Work out the finished part from the listing and answer in its coordinate system (mm). Face numbers are marked on the shaded views. A direction names the side the tool comes from. Coordinates: 2 decimals unless noted, no trailing zeros. Order: outer loops, then holes, each group sorted by start corner. A loop starts at its lowest first (then second) coordinate and runs counter-clockwise, first axis right, second up.
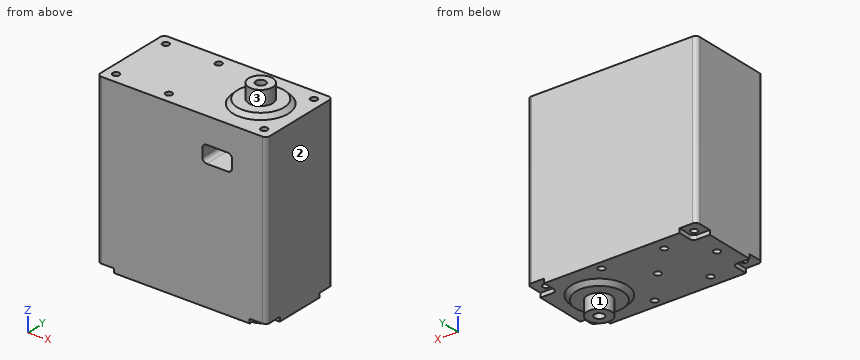
```python
from build123d import *

# Parameters (mm, degrees)
ESQUISSE1_W             = 40
ESQUISSE1_H             = 20
BOSS_EXTRU_1_DEPTH      = 40.5
ESQUISSE2_R             = 0.79
ENL_V_MAT_EXTRU_2_DEPTH = 61.334484335
ENL_V_MAT_EXTRU_3_DEPTH = 1
ESQUISSE4_R             = 0.79
ENL_V_MAT_EXTRU_4_DEPTH = 20
ESQUISSE5_R             = 6.5
BOSS_EXTRU_2_DEPTH      = 1
CHANFREIN1_SIZE         = 1
ESQUISSE6_R             = 2.85
BOSS_EXTRU_3_DEPTH      = 3.4
CONG_1_R                = 1
BOSS_EXTRU_4_START      = 1
ESQUISSE7_R             = 6.5
BOSS_EXTRU_4_DEPTH      = 1
CHANFREIN2_SIZE         = 1
BOSS_EXTRU_5_START      = 3.4
ESQUISSE8_R             = 2.85
BOSS_EXTRU_5_DEPTH      = 3.4
ENL_V_MAT_EXTRU_6_DEPTH = 15
ESQUISSE10_R            = 0.79
ENL_V_MAT_EXTRU_7_DEPTH = 20
ESQUISSE11_R            = 1.15
ENL_V_MAT_EXTRU_8_DEPTH = 15
ENL_V_START             = -15
ESQUISSE12_R            = 1.15
ENL_V_MAT_EXTRU_9_DEPTH = 15


with BuildPart() as part:
    # Esquisse1 → Boss.-Extru.1 (new body)
    with BuildSketch(Plane.XY):
        with Locations((20, 10)):
            Rectangle(ESQUISSE1_W, ESQUISSE1_H)
    extrude(amount=BOSS_EXTRU_1_DEPTH)

    # Esquisse2 → Enlèv. mat.-Extru.2 (cut, through all)
    with BuildSketch(Plane(origin=(0, 0, 0), x_dir=(-1, 0, 0), z_dir=(0, 0, -1))):
        with Locations((-2.5, 2.5)):
            Circle(ESQUISSE2_R)
        with Locations((-37.5, 2.5)):
            Circle(ESQUISSE2_R)
        with Locations((-2.5, 17.5)):
            Circle(ESQUISSE2_R)
        with Locations((-37.5, 17.5)):
            Circle(ESQUISSE2_R)
    extrude(amount=-ENL_V_MAT_EXTRU_2_DEPTH, mode=Mode.SUBTRACT)

    # Esquisse3 → Enlèv. mat.-Extru.3 (cut)
    with BuildSketch(Plane(origin=(0, 0, 0), x_dir=(-1, 0, 0), z_dir=(0, 0, -1))):
        with BuildLine():
            Line((0, 16), (-3, 16))
            ThreePointArc((-3, 16), (-3.707106781, 16.292893219), (-4, 17))
            Line((-4, 17), (-4, 20))
            Line((-4, 20), (0, 20))
            Line((0, 20), (0, 16))
        make_face()
        with BuildLine():
            Line((0, 0), (-4, 0))
            Line((-4, 0), (-4, 3))
            ThreePointArc((-4, 3), (-3.707106781, 3.707106781), (-3, 4))
            Line((-3, 4), (0, 4))
            Line((0, 4), (0, 0))
        make_face()
        with BuildLine():
            Line((-36, 0), (-40, 0))
            Line((-40, 0), (-40, 4))
            Line((-40, 4), (-37, 4))
            ThreePointArc((-37, 4), (-36.292893219, 3.707106781), (-36, 3))
            Line((-36, 3), (-36, 0))
        make_face()
        with BuildLine():
            Line((-37, 16), (-40, 16))
            Line((-40, 16), (-40, 20))
            Line((-40, 20), (-36, 20))
            Line((-36, 20), (-36, 17))
            ThreePointArc((-36, 17), (-36.292893219, 16.292893219), (-37, 16))
        make_face()
    extrude(amount=-ENL_V_MAT_EXTRU_3_DEPTH, mode=Mode.SUBTRACT)

    # Esquisse4 → Enlèv. mat.-Extru.4 (cut)
    with BuildSketch(Plane(origin=(0, 0, 0), x_dir=(-1, 0, 0), z_dir=(0, 0, -1))):
        with Locations((-3, 10)):
            Circle(ESQUISSE4_R)
        with Locations((-10, 17)):
            Circle(ESQUISSE4_R)
        with Locations((-10, 3)):
            Circle(ESQUISSE4_R)
        with Locations((-17, 10)):
            Circle(ESQUISSE4_R)
        with Locations((-24, 2)):
            Circle(ESQUISSE4_R)
        with Locations((-24, 18)):
            Circle(ESQUISSE4_R)
    extrude(amount=-ENL_V_MAT_EXTRU_4_DEPTH, mode=Mode.SUBTRACT)

    # Esquisse5 → Boss.-Extru.2 (add)
    with BuildSketch(Plane(origin=(0, 0, 0), x_dir=(-1, 0, 0), z_dir=(0, 0, -1))):
        with Locations((-30.8, 10)):
            Circle(ESQUISSE5_R)
    extrude(amount=BOSS_EXTRU_2_DEPTH)

    # Chanfrein1
    chanfrein1_edges = [part.edges().sort_by_distance(p)[0] for p in [
        (37.3, 10, -1),
    ]]
    chamfer(chanfrein1_edges, length=CHANFREIN1_SIZE - 0.0001)  # a hair under: the kernel refuses the full size

    # Esquisse6 → Boss.-Extru.3 (add)
    with BuildSketch(Plane(origin=(0, 0, -1), x_dir=(-1, 0, 0), z_dir=(0, 0, -1))):
        with Locations((-30.8, 10)):
            Circle(ESQUISSE6_R)
    extrude(amount=BOSS_EXTRU_3_DEPTH)

    # Congé1
    cong_1_edges = [part.edges().sort_by_distance(p)[0] for p in [
        (0, 20, 20.75),
        (40, 20, 20.75),
        (40, 0, 20.75),
        (0, 0, 20.75),
    ]]
    fillet(cong_1_edges, radius=CONG_1_R)

    # Esquisse7 → Boss.-Extru.4 (add)
    with BuildSketch(Plane.XY.offset(40.5).offset(BOSS_EXTRU_4_START)):
        with Locations(Location((30.8, 10, 0), (0, 0, 180))):
            Circle(ESQUISSE7_R)
    extrude(amount=-BOSS_EXTRU_4_DEPTH)

    # Chanfrein2
    chanfrein2_edges = [part.edges().sort_by_distance(p)[0] for p in [
        (37.3, 10, 41.5),
    ]]
    chamfer(chanfrein2_edges, length=CHANFREIN2_SIZE - 0.0001)  # a hair under: the kernel refuses the full size

    # Esquisse8 → Boss.-Extru.5 (add)
    with BuildSketch(Plane.XY.offset(41.5).offset(BOSS_EXTRU_5_START)):
        with Locations(Location((30.8, 10, 0), (0, 0, 180))):
            Circle(ESQUISSE8_R)
    extrude(amount=-BOSS_EXTRU_5_DEPTH)

    # Esquisse9 → Enlèv. mat.-Extru.6 (cut)
    with BuildSketch(Plane.XZ):
        with BuildLine():
            Line((30.852193658, 30.389388186), (25.852193658, 30.389388186))
            ThreePointArc((25.852193658, 30.389388186), (25.145086877, 30.682281405), (24.852193658, 31.389388186))
            Line((24.852193658, 31.389388186), (24.852193658, 33.389388186))
            ThreePointArc((24.852193658, 33.389388186), (25.145086877, 34.096494967), (25.852193658, 34.389388186))
            Line((25.852193658, 34.389388186), (30.852193658, 34.389388186))
            ThreePointArc((30.852193658, 34.389388186), (31.559300439, 34.096494967), (31.852193658, 33.389388186))
            Line((31.852193658, 33.389388186), (31.852193658, 31.389388186))
            ThreePointArc((31.852193658, 31.389388186), (31.559300439, 30.682281405), (30.852193658, 30.389388186))
        make_face()
    extrude(amount=-ENL_V_MAT_EXTRU_6_DEPTH, mode=Mode.SUBTRACT)

    # Esquisse10 → Enlèv. mat.-Extru.7 (cut)
    with BuildSketch(Plane.XY.offset(40.5)):
        with Locations((15, 2.5)):
            Circle(ESQUISSE10_R)
        with Locations((15, 17.5)):
            Circle(ESQUISSE10_R)
    extrude(amount=-ENL_V_MAT_EXTRU_7_DEPTH, mode=Mode.SUBTRACT)

    # Esquisse11 → Enlèv. mat.-Extru.8 (cut)
    with BuildSketch(Plane.XY.offset(44.9)):
        with Locations((30.8, 10)):
            Circle(ESQUISSE11_R)
    extrude(amount=-ENL_V_MAT_EXTRU_8_DEPTH, mode=Mode.SUBTRACT)

    # Esquisse12 → Enlèv. mat.-Extru.9 (cut)
    with BuildSketch(Plane(origin=(0, 0, -4.4), x_dir=(-1, 0, 0), z_dir=(0, 0, -1)).offset(ENL_V_START)):
        with Locations(Location((-30.8, 10, 0), (0, 0, 180))):
            Circle(ESQUISSE12_R)
    extrude(amount=ENL_V_MAT_EXTRU_9_DEPTH, mode=Mode.SUBTRACT)


solid = part.part
```
1. Flat-ended cylindrical pins translate along their axes: pin 1 (10 mm diameter, centred on x = 20, z = 6, fed in from -Y); pin 2 (0.5 mm diameter, centred on x = 2, z = 0.5, fed in from +Y); pin 3 (0.8 mm diameter, centred on x = 10, y = 17, fed in from -Z); pin 4 (2.5 mm diameter, centred on x = 10, y = 17, fed in from -Z). Find the tip coordinate at first contact, or state that the pin passes through.
2. Consider probe 1 along Y at (x, z) = (2.5, 28.5); probe 2 along Y at (x, z) = (24, 11.5); probe 3 along Y at (x, z) = (30.8, 7.5). Determine where each line is inside the solid, lowest interval first.
3. The part is cut by section C-C (x = 6). Determine the outline of the cut face in (y, z), plus the area to 3 significant figures.
4. The part is cut by section A-A (z = 2). Count the separate pieces of the cut face and the enclosed holes in it, plus the area to 3 significant figures.
5. For the marked faces 1, 2 and 3, determine the directions among +Z, -Z, +X, -X, +Y, -Y from which every point of the face is accessible in a straight line to the end or side of a thin tool.
6. The part is cut by section B-B (x = 15). Determine the outline of the cut face in (y, z), plus the area to 3 significant figures.
Worked out:
1. pin 1: stops at y = 0
1. pin 2: stops at y = 16
1. pin 3: stops at z = 20
1. pin 4: stops at z = 0
2. probe 1: y = 0 to 1.71, 3.29 to 16.71, 18.29 to 20
2. probe 2: y = 0 to 1.21, 2.79 to 17.21, 18.79 to 20
2. probe 3: y = 0 to 8.85, 11.15 to 20
3. outline: (0, 0) - (20, 0) - (20, 40.5) - (0, 40.5) - close
3. area: 810 mm2
4. separate pieces: 1
4. enclosed holes: 11
4. area: 775 mm2
5. face 1: -Z
5. face 2: +Z, -Z, +X, +Y, -Y
5. face 3: +Z
6. outline: (0, 0) - (20, 0) - (20, 40.5) - (18.29, 40.5) - (18.29, 20.5) - (16.71, 20.5) - (16.71, 40.5) - (3.29, 40.5) - (3.29, 20.5) - (1.71, 20.5) - (1.71, 40.5) - (0, 40.5) - close
6. area: 747 mm2
